Input: dimensioned drawing with shaded views. Units: mm. Origin: part minimum x, y, z. A direction names the side the tool comes from. Round coordinates to 2 decimals unless told otherwise and drop trailing zeros. Order: outer loops, then holes, each group sorted by start corner. A loop starts at its lowest first (then second) coordinate and runs counter-clockwise, first axis right, second up. Notation, with made-up numbers: M 18.5,-17 L 47.5,-17 A29 cw 47.5,20 Z; hole C -15.5,-14.75 d3. An arc over 180 degrees is marked long. One line per question, with ' | ' between items.
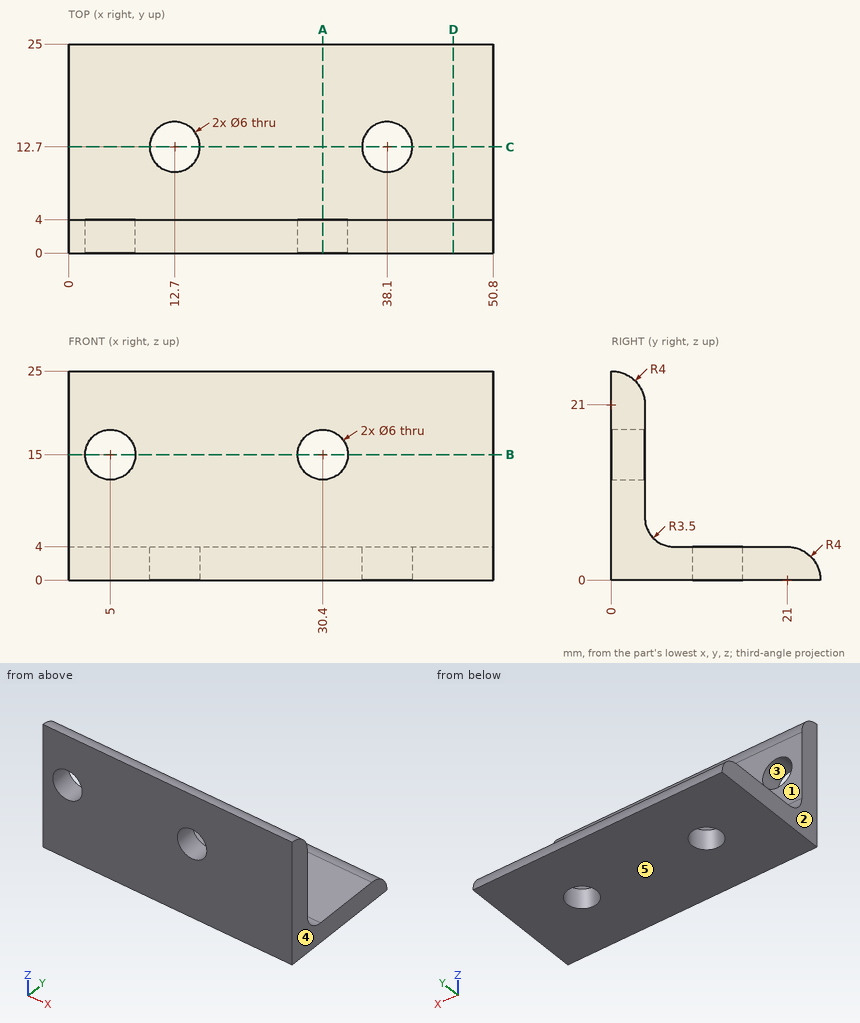
Item 1: Access query for the marked faces 1 and 2. Directions: +Z, -Z, +X, -X, +Y, -Y. A direction counts if a zero-diameter tool reaches every point of the face in a straight line with its end or side. Return the directions, or none.
Report:
face 1: +Z, +X, -X, +Y | face 2: +Z, -Z, -X, +Y, -Y
Item 2: Section query C-C, the plane y = 12.7. Return loops of the section in (x, z), plus the area to 3 significant figures.
Report:
outline: M 0,0 L 9.7,0 L 9.7,4 L 0,4 Z; M 15.7,0 L 35.1,0 L 35.1,4 L 15.7,4 Z; M 41.1,0 L 50.8,0 L 50.8,4 L 41.1,4 Z | area: 155 mm²
Item 3: Line query: line 1 along X through (y, z) = (2.85, 15); line 2 along Z through (x, y) = (42, 10). Output: solid intervals per line, ascending. Write a range as from..to.
Report:
line 1: 0..2, 8..27.4, 33.4..50.8 | line 2: 0..4
Item 4: Section query D-D, the plane x = 46. Return loops of the section in (y, z), plus the area to 3 significant figures.
Report:
outline: M 0,0 L 25,0 A4 ccw 21,4 L 7.5,4 A3.5 cw 4,7.5 L 4,21 A4 ccw 0,25 Z | area: 180 mm²
Item 5: First-contact query: pin 1 (1.5 mm diameter, centred on x = 38.5, z = 10.5, fed in from +Y); pin 2 (9.5 mm diameter, centred on x = 38.1, y = 12.7, fed in from +Z); pin 3 (5 mm diameter, centred on x = 33, y = 6, fed in from +Z). Flat tips, straight axial feed; report the tip coordinate or a pass-through.
Report:
pin 1: y = 4 | pin 2: z = 4 | pin 3: z = 22.94
Item 6: Section query B-B, the plane z = 15. Return loops of the section in (x, y), plus the area to 3 significant figures.
Report:
outline: M 0,0 L 2,0 L 2,4 L 0,4 Z; M 8,0 L 27.4,0 L 27.4,4 L 8,4 Z; M 33.4,0 L 50.8,0 L 50.8,4 L 33.4,4 Z | area: 155 mm²
Item 7: Section query A-A, the plane x = 30.4. Return loops of the section in (y, z), plus the area to 3 significant figures.
Report:
outline: M 0,0 L 25,0 A4 ccw 21,4 L 7.5,4 A3.5 cw 4,7.5 L 4,12 L 0,12 Z; M 0,18 L 4,18 L 4,21 A4 ccw 0,25 Z | area: 156 mm²
Item 8: Mould query, pull axis X, two halves, no side actions, for the marked faces 3, 4 and 5. Classes: +X half, -X half, draft (parallel to the pull), parting line (faces both ways), or undercut.
Report:
face 3: undercut | face 4: +X half | face 5: draft
